Solid Edge part; units mm, degrees
sketch "Sketch1" plane through (0, 0, 0) normal (0, 0, 1) x (1, 0, 0)
  circle A0 centre (0, 0) radius 4.25
extrude "Protrusion1" add sketch "Sketch1" along normal blind 5
sketch "Sketch2" plane through (0, 0, 0) normal (0, 0, -1) x (1, 0, 0)
  circle A0 centre (0, 0) radius 2.5
extrude "Protrusion2" add sketch "Sketch2" along normal blind 30
sketch "Sketch3" plane through (0, 0, -30) normal (0, 0, -1) x (1, 0, 0)
  circle A0 centre (0, 0) radius 2.4997
extrude "Cutout1" cut sketch "Sketch3" against normal blind 22 flip side to cut
chamfer "Chamfer_1" distance 0.375 angle 45 1 edges at (-2.4997, 0, -30)
sketch "Sketch4" plane through (0, 0, 5) normal (0, 0, 1) x (1, 0, 0)
  line L0 (-1.1547, 2) -> (1.1547, 2)
  line L1 (2.3094, 0) -> (1.1547, 2)
  line L2 (1.1547, -2) -> (2.3094, 0)
  line L3 (-1.1547, -2) -> (1.1547, -2)
  line L4 (-2.3094, 0) -> (-1.1547, -2)
  line L5 (-1.1547, 2) -> (-2.3094, 0)
extrude "Cutout2" cut sketch "Sketch4" against normal blind 2.5
properties part number "185701" material "Stainless Steel, 304"
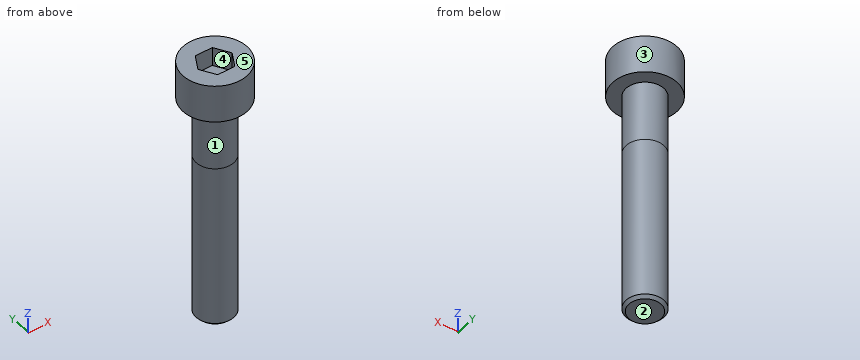
Verification items for the finished model (mm, model axes). Face numbers are marked on the shaded views. A direction names the side the tool comes from. Give positions to 0.01 mm unless a question says otherwise; leave off trailing zeros. Write each loop counter-clockwise with the first axis right and the second up, starting at its lowest first coordinate (ties: lowest second). Pieces come first, ordered by that corner, then holes. Notation, with made-up numbers: (31.5, -36.75) - (48.5, -36.75) arc R27 ccw to (48.5, -8.75) - close; hole circle Ø3 at (30.25, -31). An arc over 180 degrees is marked (long way). Answer as CSV lines item,"result". Start each with the question number.
1. Draft check along Y on the marked faces 3, 4 and 5. Enter one of: pulls with the +Y half, pulls with the -Y half, needs draft (parallel to the pull), parting line crosses it, or undercut.
2. Sectioned sample at B-B (z = -17.5). Record the boundary of the cut face in (x, y).
3. Sectioned sample at C-C (x = 3.25). Record the boundary of the cut face in (y, z).
4. Set-up check for the marked faces 1 and 2: record each of +Z, -Z, +X, -X, +Y, -Y from which the full face is reachable in a straight line by a thin tool's end or side.
5. Depth check by flat-ended pin: pin 1 (1.5 mm diameter, centred on y = -2.5, z = -26, fed in from -X); pin 2 (0.7 mm diameter, centred on x = -0.5, z = 4, fed in from -Y); pin 3 (3 mm diameter, centred on y = 0.5, z = -14, fed in from +X). Enter the tip coordinate at first touch or a pass-through.
6. Thickness scan on line 1 (Z direction, x = 0, y = 1.5); line 2 (Y direction, x = 1.5, z = -2); line 3 (Y direction, x = 0, z = -23). Record the ranges inside material, lowest first.
Derived:
1,face 3,"parting line crosses it"
1,face 4,"undercut"
1,face 5,"needs draft"
2,outline,"circle Ø5 at (0, 0)"
3,outline,"(-2.74, 0) - (2.74, 0) - (2.74, 5) - (-2.74, 5) - close"
4,face 1,"-Z"
4,face 2,"-Z, +X, -X, +Y, -Y"
5,pin 1,"x = -1.78"
5,pin 2,"y = -4.25"
5,pin 3,"x = 2.5"
6,line 1,"-30 to 2.5"
6,line 2,"-2 to 2"
6,line 3,"-2.5 to 2.5"
